```python
from build123d import *

# Parameters (mm, degrees)
BOX015_W     = 3.25
BOX015_H     = 3
BOX015_DEPTH = 4
BOX014_W     = 3.25
BOX014_H     = 3
BOX014_DEPTH = 4
BOX013_W     = 8
BOX013_H     = 4
BOX013_DEPTH = 5


with BuildPart() as cubo015:
    # Box015 → Box015 (new body)
    with BuildSketch(Plane(origin=(10.25, 2.5, -5), x_dir=(1, 0, 0), z_dir=(0, 0, 1))):
        with Locations((1.625, 1.5)):
            Rectangle(BOX015_W, BOX015_H)
    extrude(amount=BOX015_DEPTH)


with BuildPart() as cubo014:
    # Box014 → Box014 (new body)
    with BuildSketch(Plane(origin=(6.5, 2.5, -5), x_dir=(1, 0, 0), z_dir=(0, 0, 1))):
        with Locations((1.625, 1.5)):
            Rectangle(BOX014_W, BOX014_H)
    extrude(amount=BOX014_DEPTH)


with BuildPart() as obj1:
    # Box013 → Box013 (new body)
    with BuildSketch(Plane(origin=(6, 2, -5), x_dir=(1, 0, 0), z_dir=(0, 0, 1))):
        with Locations((4, 2)):
            Rectangle(BOX013_W, BOX013_H)
    extrude(amount=BOX013_DEPTH)

    # Cut009: cut Cubo014
    add(cubo014.part, mode=Mode.SUBTRACT)

    # Cut010: cut Cubo015
    add(cubo015.part, mode=Mode.SUBTRACT)


with BuildPart() as obj1_1:
    # Cut010 placement: moved
    add(obj1.part.moved(Location((0, 0, 0.4))))


solid = obj1_1.part
```
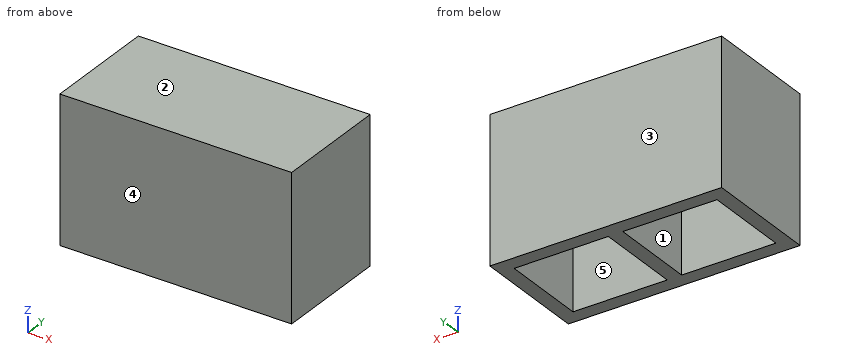
Here's how the part is built. I have some questions about the finished solid (model axes, mm). Face numbers are marked on the shaded views. A direction names the side the tool comes from. Coordinates: 2 decimals unless noted, no trailing zeros. Loops run counter-clockwise (first coordinate to the right, second up) from the corner with the lowest first, then second, coordinate; pieces in that order, holes last. Notation, with made-up numbers: (25.25, 87) - (33.25, 87) arc R14 ccw to (33.25, 108) - close; hole circle Ø8 at (-8, -16.75). An arc over 180 degrees is marked (long way). Answer as CSV lines item,"result".
Q1. If I drill on L1, parallel to X at y = 3.7, z = -4; L2, parallel to Y at x = 11.25, z = -2.7; L3, parallel to Z at x = 7.5, y = 5.05, over which ranges is the centre line in solid material (lowest first)? Write a range as [from, to].
Response:
L1,"[6, 6.5], [9.75, 10.25], [13.5, 14]"
L2,"[2, 2.5], [5.5, 6]"
L3,"[-0.6, 0.4]"
Q2. For the marked faces 4 and 5, which set-ups out of +Z, -Z, +X, -X, +Y, -Y let a thin tool reach every point of the face, with its end or its side?
Response:
face 4,"+Z, -Z, +X, -X, -Y"
face 5,"-Z"
Q3. If we section it at B-B, the plane x = 11.25: Write out the boundary of the cut face in (y, z), and give its area (3 significant figures).
Response:
outline,"(2, -4.6) - (2.5, -4.6) - (2.5, -0.6) - (5.5, -0.6) - (5.5, -4.6) - (6, -4.6) - (6, 0.4) - (2, 0.4) - close"
area,"8.00 mm2"
Q4. We'd pull the mould along Y, two halves only. Please class the marked faces 1, 2 and 3: pulls with the +Y half, pulls with the -Y half, needs draft (parallel to the pull), parting line crosses it, or undercut.
Response:
face 1,"undercut"
face 2,"needs draft"
face 3,"pulls with the +Y half"
Q5. If we section it at C-C, the plane y = 3.2: Write out the boundary of the cut face in (x, z), and give its area (3 significant figures).
Response:
outline,"(6, -4.6) - (6.5, -4.6) - (6.5, -0.6) - (9.75, -0.6) - (9.75, -4.6) - (10.25, -4.6) - (10.25, -0.6) - (13.5, -0.6) - (13.5, -4.6) - (14, -4.6) - (14, 0.4) - (6, 0.4) - close"
area,"14.0 mm2"
Q6. If we section it at A-A, the plane z = -2.5: Write out the boundary of the cut face in (x, y), and give its area (3 significant figures).
Response:
outline,"(6, 2) - (14, 2) - (14, 6) - (6, 6) - close; hole (6.5, 2.5) - (9.75, 2.5) - (9.75, 5.5) - (6.5, 5.5) - close; hole (10.25, 2.5) - (13.5, 2.5) - (13.5, 5.5) - (10.25, 5.5) - close"
area,"12.5 mm2"
